The model under review builds one solid part; all positions refer to its coordinate system, in mm. Face numbers are marked on the shaded views. A direction names the side the tool comes from. Coordinates: 2 decimals unless noted, no trailing zeros. Loops run counter-clockwise (first coordinate to the right, second up) from the corner with the lowest first, then second, coordinate; pieces in that order, holes last. Notation, with made-up numbers: (26.5, 9.25) - (78.5, 9.25) arc R12 cw to (78.5, 22.25) - close; hole circle Ø8 at (-2, 62.25). An arc over 180 degrees is marked (long way). Answer in a Markdown table with one row per item. Add a question column.
(1) We need section A-A on x = 0. Write out the cut boundary in (y, z).
(2) We need section D-D on x = 12. Write out the cut boundary in (y, z), plus the area to 3 significant figures.
(3) We need section B-B on y = 6. Write out the cut boundary in (x, z), plus the area to 3 significant figures.
(4) For line 1 along X through (y, z) = (0, -7.25); line 2 along Y through (x, z) = (-7.75, -5); line 3 along Y through (x, z) = (7, -6), list the stretches that pass through material, from the lowest coordinate up.
(5) Machinability: for the marked faces 1, 2 and 3, which of the approach directions +Z, -Z, +X, -X, +Y, -Y give a long, thin tool a straight path to every point of the face, cutting with its end or side? Answer none if there is none.
(6) We need section C-C on z = -9. Write out the cut boundary in (x, y), plus the area to 3 significant figures.
(7) For P1, Ø2, axis at y = 12, z = -46.5, coming from the +X side; P2, Ø1.5, axis at y = -1, z = -48, coming from the -X side; P3, Ø3, axis at y = -5.5, z = -28.5, coming from the +X side, all flat-tipped, find the tip position at first contact; note any pin that passes through.
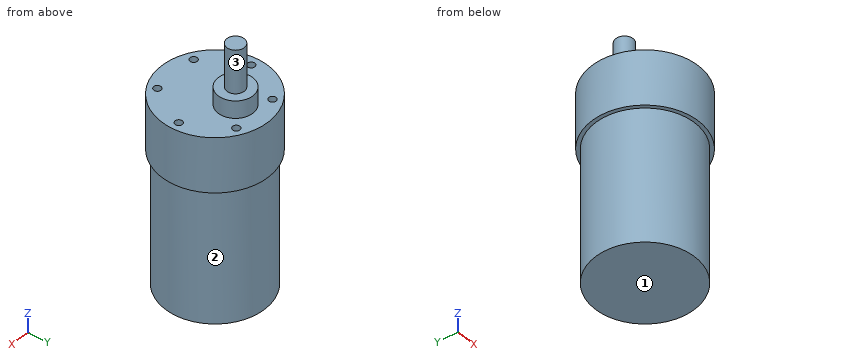
from build123d import *

# Parameters (mm, degrees)
SKETCH4_R                       = 6
BOSS_EXTRUDE3_DEPTH             = 6
SKETCH4_3_R                     = 3
BOSS_EXTRUDE4_DEPTH             = 21
TAP_DRILL_FOR_M3X0_5_TAP1_D     = 2.5
TAP_DRILL_FOR_M3X0_5_TAP1_DEPTH = 10
TAP_DRILL_FOR_M3X0_5_TAP1_TIP   = 0.751075774


with BuildPart() as part:
    # Sketch3 → Revolve1 (revolve)
    with BuildSketch(Plane(origin=(0, 0, 0), x_dir=(0, 0, -1), z_dir=(1, 0, 0))):
        Polygon((0, 0), (0, 18.5), (19, 18.5), (19, 17.25), (49.8, 17.25), (65.1, 17.25), (65.1, 0), align=None)
    revolve(axis=Axis((0, 0, 4.918404278), (0, 0, -1)))

    # Sketch4 → Boss-Extrude3 (add)
    with BuildSketch(Plane.XY):
        with Locations((0, 7)):
            Circle(SKETCH4_R)
    extrude(amount=BOSS_EXTRUDE3_DEPTH)

    # Sketch4<3> → Boss-Extrude4 (add)
    with BuildSketch(Plane.XY):
        with Locations((0, 7)):
            Circle(SKETCH4_3_R)
    extrude(amount=BOSS_EXTRUDE4_DEPTH)

    # Tap Drill for M3x0.5 Tap1
    with Locations(Plane.XY):
        with Locations((-15.5, 0), (-7.75, 13.423393759), (7.75, 13.423393759), (15.5, 0), (7.75, -13.423393759), (-7.75, -13.423393759)):
            Hole(TAP_DRILL_FOR_M3X0_5_TAP1_D / 2, depth=TAP_DRILL_FOR_M3X0_5_TAP1_DEPTH)
            with Locations((0, 0, -(TAP_DRILL_FOR_M3X0_5_TAP1_DEPTH + TAP_DRILL_FOR_M3X0_5_TAP1_TIP / 2))):  # 118° drill point
                Cone(0, TAP_DRILL_FOR_M3X0_5_TAP1_D / 2, TAP_DRILL_FOR_M3X0_5_TAP1_TIP, mode=Mode.SUBTRACT)


solid = part.part
Outcome:
| question | item | result |
|---|---|---|
| 1 | outline | (-18.5, -19) - (-17.25, -19) - (-17.25, -65.1) - (17.25, -65.1) - (17.25, -19) - (18.5, -19) - (18.5, 0) - (13, 0) - (13, 6) - (10, 6) - (10, 21) - (4, 21) - (4, 6) - (1, 6) - (1, 0) - (-18.5, 0) - close |
| 2 | outline | (-14.08, -19) - (-12.39, -19) - (-12.39, -65.1) - (12.39, -65.1) - (12.39, -19) - (14.08, -19) - (14.08, 0) - (-14.08, 0) - close |
| 2 | area | 1,680 mm² |
| 3 | outline | (-17.5, -19) - (-16.17, -19) - (-16.17, -65.1) - (16.17, -65.1) - (16.17, -19) - (17.5, -19) - (17.5, 0) - (5.92, 0) - (5.92, 6) - (2.83, 6) - (2.83, 21) - (-2.83, 21) - (-2.83, 6) - (-5.92, 6) - (-5.92, 0) - (-17.5, 0) - close |
| 3 | area | 2,310 mm² |
| 4 | line 1 | -18.5 to -16.75, -14.25 to 14.25, 16.75 to 18.5 |
| 4 | line 2 | -16.8 to -14.67, -12.17 to 12.17, 14.67 to 16.8 |
| 4 | line 3 | -17.12 to -14.42, -12.42 to 12.42, 14.42 to 17.12 |
| 5 | face 1 | -Z, +X, -X, +Y, -Y |
| 5 | face 2 | -Z |
| 5 | face 3 | +Z |
| 6 | outline | circle Ø37 at (0, 0); hole circle Ø2.5 at (-15.5, 0); hole circle Ø2.5 at (-7.75, -13.42); hole circle Ø2.5 at (-7.75, 13.42); hole circle Ø2.5 at (7.75, -13.42); hole circle Ø2.5 at (7.75, 13.42); hole circle Ø2.5 at (15.5, 0) |
| 6 | area | 1,050 mm² |
| 7 | P1 | x = 13.29 |
| 7 | P2 | x = -17.25 |
| 7 | P3 | x = 16.78 |
